Read the model definition and answer for the solid it produces. Units are mm, in the model's axes. Face numbers are marked on the shaded views. A direction names the side the tool comes from. Coordinates: 2 decimals unless noted, no trailing zeros. Order: outer loops, then holes, each group sorted by start corner. A loop starts at its lowest first (then second) coordinate and runs counter-clockwise, first axis right, second up. Notation, with made-up numbers: (41, 13.5) -> (61, 13.5) arc R20 cw to (61, 32.5) -> close; hole circle Ø8 at (24.25, -28). An arc over 180 degrees is marked (long way). Answer as a JSON object with one key per item and string values. Group by question number.
1) Section B-B on x = -34 is taken. Determine the outline of the cut face in (y, z), and give its area (3 significant figures).
2) Determine the mould class of the marked faces 3, 4 and 5 for opening direction Y: released by +Y, released by -Y, zero draft, split by the parting line, or undercut.
3) Consider L1, parallel to Y at x = 39.5, z = 59; L2, parallel to Z at x = 45, y = -38.5; L3, parallel to X at y = -15.5, z = 52.5. Determine where each line is inside the solid, lowest interval first.
4) A tool of negligible diameter and unlimited length cuts with its end or side. For the marked faces 1 and 2, from which of +Z, -Z, +X, -X, +Y, -Y can it reach the whole face along a straight path? Write none if from no direction.
5) Section A-A on y = -30 is taken. Determine the outline of the cut face in (x, z), and give its area (3 significant figures).
6) Section D-D on z = 14.5 is taken. Determine the outline of the cut face in (x, y), and give its area (3 significant figures).
7) Given pin 1 (2 mm diameter, centred on x = 63.5, y = -36.5, fed in from -Z); pin 2 (6 mm diameter, centred on x = -49, y = 33, fed in from +Z); pin 3 (6 mm diameter, centred on y = 16, z = 49, fed in from -X), each flat-ended and moving along its own axis, determine where each tip first touches the part or whether it passes through.
8) Section C-C on z = 36 is taken. Determine the outline of the cut face in (x, y).
from build123d import *

# Parameters (mm, degrees)
F0_W     = 130
F0_H     = 110
F1_DEPTH = 75
F3_DEPTH = 110
F4_T     = -4.5
F6_DEPTH = 110.001
F7_W     = 20
F7_H     = 20
F8_DEPTH = 4.5


with BuildPart() as f1:
    # F0 (on Top) → F1 (new body)
    with BuildSketch(Plane.XY):
        Rectangle(F0_W, F0_H)
    extrude(amount=F1_DEPTH)

    # F2 (on face) → F3 (join, through all)
    with BuildSketch(Plane.XZ.offset(55)):
        Polygon((-85.096189, 75), (-65, 0), (-65, 75), align=None)
    extrude(amount=-F3_DEPTH)

    # F4
    f4_openings = [f1.faces().sort_by_distance(p)[0] for p in [
        (-10.048095, 0, 75),
    ]]
    offset(amount=F4_T, openings=f4_openings)

    # F5 (on face) → F6 (cut, through all)
    with BuildSketch(Plane.XZ.offset(55)):
        Polygon((-80.316136, 57.160596), (-42.05941, 75), (-85.419632, 75), align=None)
    extrude(amount=-F6_DEPTH, mode=Mode.SUBTRACT)

    # F7 (on face) → F8 (cut, through all)
    with BuildSketch(Plane.YZ.offset(65)):
        with Locations((-35, 58)):
            Rectangle(F7_W, F7_H)
        with Locations((35, 58)):
            Rectangle(F7_W, F7_H)
    extrude(amount=-F8_DEPTH, mode=Mode.SUBTRACT)


solid = f1.part
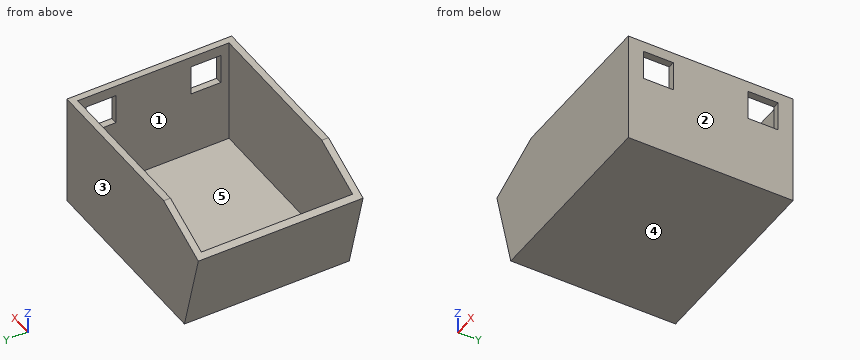
Worked answers:
{
 "1": {"outline": "(-55, 0) -> (55, 0) -> (55, 75) -> (50.5, 75) -> (50.5, 4.5) -> (-50.5, 4.5) -> (-50.5, 75) -> (-55, 75) -> close", "area": "1,130 mm²"},
 "2": {"face 3": "released by +Y", "face 4": "zero draft", "face 5": "undercut"},
 "3": {"L1": "y = -55 to -50.5, 50.5 to 55", "L2": "z = 0 to 4.5", "L3": "x = -79.07 to -74.41, 60.5 to 65"},
 "4": {"face 1": "+Z", "face 2": "+Z, -Z, +X, +Y, -Y"},
 "5": {"outline": "(-80.32, 57.16) -> (-65, 0) -> (65, 0) -> (65, 48) -> (60.5, 48) -> (60.5, 4.5) -> (-61.55, 4.5) -> (-76.17, 59.09) -> close; (60.5, 68) -> (65, 68) -> (65, 75) -> (60.5, 75) -> close", "area": "1,060 mm²"},
 "6": {"outline": "(-68.89, -55) -> (65, -55) -> (65, 55) -> (-68.89, 55) -> close; hole (-64.23, -50.5) -> (60.5, -50.5) -> (60.5, 50.5) -> (-64.23, 50.5) -> close", "area": "2,130 mm²"},
 "7": {"pin 1": "stops at z = 0", "pin 2": "stops at z = 4.5", "pin 3": "stops at x = -78.93"},
 "8": {"outline": "(-74.65, -55) -> (65, -55) -> (65, 55) -> (-74.65, 55) -> close; hole (-69.99, -50.5) -> (60.5, -50.5) -> (60.5, 50.5) -> (-69.99, 50.5) -> close"}
}
